Geometry check sheet. Reference: the model listing, model coordinates, mm. Face numbers are marked on the shaded views. A direction names the side the tool comes from. Round coordinates to 2 decimals unless told otherwise and drop trailing zeros. Order: outer loops, then holes, each group sorted by start corner. A loop starts at its lowest first (then second) coordinate and runs counter-clockwise, first axis right, second up.
(1) Release check for a two-part mould opening along Y. For the marked faces 4, 5 and 6 record: +Y half, -Y half, draft (parallel to the pull), parting line (faces both ways), or undercut.
(2) Material ranges on line 1 along X through (y, z) = (1.55, 10); line 2 along Z through (x, y) = (58, 1.95); line 3 along X through (y, z) = (46.5, 11), recorded low to high.
(3) Go/stop test with flat-tipped pins: pin 1 (5 mm diameter, centred on x = 52.5, z = 7, fed in from +Y); pin 2 (3.5 mm diameter, centred on y = 78.5, z = 10, fed in from +X); pin 3 (3.5 mm diameter, centred on y = 78.5, z = 11, fed in from -X). Record where each tip stops, or that it passes through.
(4) Sectioned sample at B-B (x = 58). Record the boundary of the cut face in (y, z).
(5) Sectioned sample at D-D (x = 34). Record the boundary of the cut face in (y, z).
(6) Set-up check for the marked faces 1, 2 and 3: record each of +Z, -Z, +X, -X, +Y, -Y from which the full face is reachable in a straight line by a thin tool's end or side.
(7) Sectioned sample at A-A (z = 13). Record the boundary of the cut face in (x, y), plus the area to 3 significant figures.
(8) Sectioned sample at C-C (z = 18.5). Record the boundary of the cut face in (x, y).
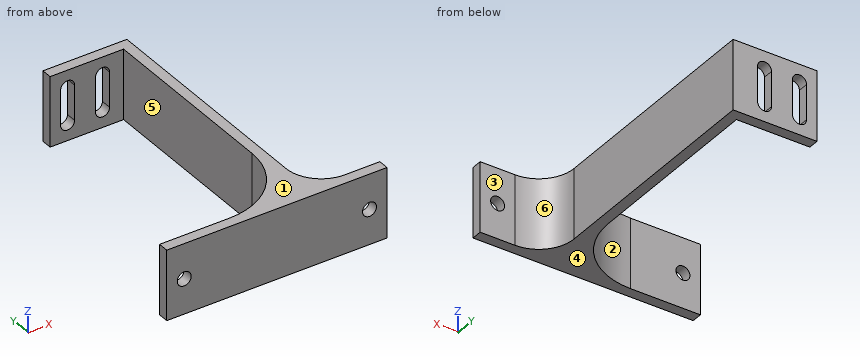
from build123d import *

# Parameters (mm, degrees)
BOSS_EXTRU_1_DEPTH      = 20
ENL_V_MAT_EXTRU_1_DEPTH = 3
CONG_1_R                = 20
CONG_2_R                = 10
ESQUISSE3_R             = 2
ENL_V_MAT_EXTRU_2_DEPTH = 3


with BuildPart() as part:
    # Esquisse1 → Boss.-Extru.1 (new body)
    with BuildSketch(Plane.XY):
        Polygon((43, 3), (63, 3), (63, 0), (0, 0), (0, 3), (40, 3), (40, 77), (19, 77), (19, 80), (43, 80), align=None)
    extrude(amount=BOSS_EXTRU_1_DEPTH)

    # Esquisse2 → Enlèv. mat.-Extru.1 (cut)
    with BuildSketch(Plane(origin=(0, 80, 0), x_dir=(1, 0, 0), z_dir=(0, 1, 0))):
        with BuildLine():
            Line((26, -5), (26, -15))
            ThreePointArc((26, -15), (24, -17), (22, -15))
            Line((22, -15), (22, -5))
            ThreePointArc((22, -5), (24, -3), (26, -5))
        make_face()
        with BuildLine():
            Line((36, -5), (36, -15))
            ThreePointArc((36, -15), (34, -17), (32, -15))
            Line((32, -15), (32, -5))
            ThreePointArc((32, -5), (34, -3), (36, -5))
        make_face()
    extrude(amount=-ENL_V_MAT_EXTRU_1_DEPTH, mode=Mode.SUBTRACT)

    # Congé1
    cong_1_edges = [part.edges().sort_by_distance(p)[0] for p in [
        (40, 3, 10),
    ]]
    fillet(cong_1_edges, radius=CONG_1_R)

    # Congé2
    cong_2_edges = [part.edges().sort_by_distance(p)[0] for p in [
        (43, 3, 10),
    ]]
    fillet(cong_2_edges, radius=CONG_2_R)

    # Esquisse3 → Enlèv. mat.-Extru.2 (cut)
    with BuildSketch(Plane(origin=(0, 3, 0), x_dir=(1, 0, 0), z_dir=(0, 1, 0))):
        with Locations((5, -10)):
            Circle(ESQUISSE3_R)
        with Locations((58, -10)):
            Circle(ESQUISSE3_R)
    extrude(amount=-ENL_V_MAT_EXTRU_2_DEPTH, mode=Mode.SUBTRACT)


solid = part.part
Answer below:
1. face 4: draft
1. face 5: undercut
1. face 6: +Y half
2. line 1: x = 0 to 3, 7 to 56, 60 to 63
2. line 2: z = 0 to 8, 12 to 20
2. line 3: x = 40 to 43
3. pin 1: stops at y = 3.46
3. pin 2: stops at x = 43
3. pin 3: stops at x = 19
4. outline: (0, 0) - (3, 0) - (3, 8) - (0, 8) - close; (0, 12) - (3, 12) - (3, 20) - (0, 20) - close
5. outline: (0, 0) - (8.72, 0) - (8.72, 20) - (0, 20) - close; (77, 0) - (80, 0) - (80, 3) - (77, 3) - close; (77, 17) - (80, 17) - (80, 20) - (77, 20) - close
6. face 1: +Z, +X, -X, +Y, -Y
6. face 2: +Z, -Z, -X
6. face 3: +Z, -Z, +X, +Y
7. outline: (0, 0) - (63, 0) - (63, 3) - (53, 3) arc R10 cw to (43, 13) - (43, 80) - (36, 80) - (36, 77) - (40, 77) - (40, 23) arc R20 cw to (20, 3) - (0, 3) - close; (19, 77) - (22, 77) - (22, 80) - (19, 80) - close; (26, 77) - (32, 77) - (32, 80) - (26, 80) - close
7. area: 566 mm2
8. outline: (0, 0) - (63, 0) - (63, 3) - (53, 3) arc R10 cw to (43, 13) - (43, 80) - (19, 80) - (19, 77) - (40, 77) - (40, 23) arc R20 cw to (20, 3) - (0, 3) - close
